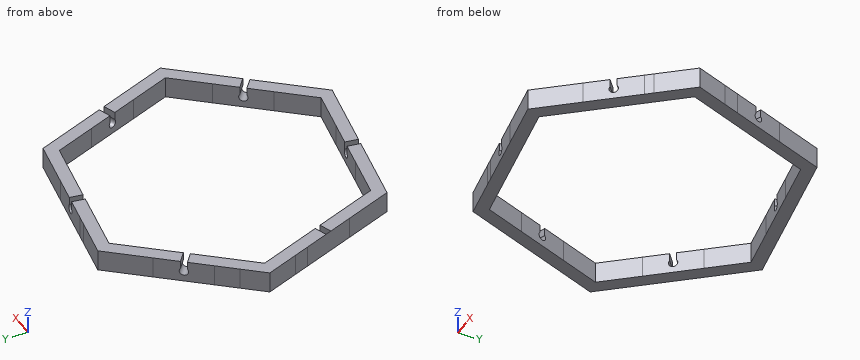
Autodesk Fusion 360 part; units mm, degrees
sketch "Sketch1" plane through (0, 0, 0) normal (0, 0, 1) x (1, 0, 0)
  line L0 (-10.798, 13.3938) -> (-13.526, 20.8958)
  line L1 (-9.4934, 25.6987) -> (-13.526, 20.8958)
  line L2 (19.2845, 47.1681) -> (9.9209, 48.822)
  line L3 (55.6112, 15.5789) -> (58.2905, 8.2107)
  line L4 (52.0708, 0.8027) -> (58.2905, 8.2107)
  line L5 (8.3931, -15.0435) -> (-1.0646, -13.373)
  line L6 (-10.798, 13.3938) -> (-9.5166, 9.87)
  line L7 (-5.074, -2.3473) -> (-1.0646, -13.373)
  line L8 (1.1628, -10.72) -> (-2.2546, -1.322)
  line L9 (-6.6972, 10.8953) -> (-10.1147, 20.2932)
  line L10 (33.6598, -16.4599) -> (23.8122, -14.7206)
  line L11 (11.0104, -12.4594) -> (1.1628, -10.72)
  line L12 (8.3931, -15.0435) -> (10.4886, -15.4136)
  line L13 (23.2904, -17.6748) -> (34.8436, -19.7155)
  line L14 (54.8793, 8.8133) -> (48.4491, 1.1547)
  line L15 (40.0899, -8.8014) -> (33.6598, -16.4599)
  line L16 (52.0708, 0.8027) -> (50.7467, -0.7743)
  line L17 (42.3875, -10.7304) -> (34.8436, -19.7155)
  line L18 (43.6017, 39.8265) -> (47.0192, 30.4285)
  line L19 (51.4618, 18.2112) -> (54.8793, 8.8133)
  line L20 (55.6112, 15.5789) -> (54.2812, 19.2364)
  line L21 (49.8385, 31.4537) -> (45.8292, 42.4795)
  line L22 (11.1048, 45.5664) -> (20.9523, 43.827)
  line L23 (33.7542, 41.5658) -> (43.6017, 39.8265)
  line L24 (19.2845, 47.1681) -> (21.4741, 46.7813)
  line L25 (34.276, 44.5201) -> (45.8292, 42.4795)
  line L26 (-10.1147, 20.2932) -> (-3.6845, 27.9518)
  line L27 (4.6746, 37.9079) -> (11.1048, 45.5664)
  line L28 (-9.4934, 25.6987) -> (-5.9821, 29.8808)
  line L29 (2.3771, 39.8369) -> (9.9209, 48.822)
  line L30 (50.7467, -0.7743) -> (42.3875, -10.7304)
  line L31 (40.0899, -8.8014) -> (48.4491, 1.1547)
  line L32 (23.2904, -17.6748) -> (10.4886, -15.4136)
  line L33 (11.0104, -12.4594) -> (23.8122, -14.7206)
  line L34 (-2.2546, -1.322) -> (-6.6972, 10.8953)
  line L35 (-9.5166, 9.87) -> (-5.074, -2.3473)
  line L36 (-3.6845, 27.9518) -> (4.6746, 37.9079)
  line L37 (2.3771, 39.8369) -> (-5.9821, 29.8808)
  line L38 (20.9523, 43.827) -> (33.7542, 41.5658)
  line L39 (34.276, 44.5201) -> (21.4741, 46.7813)
  line L40 (49.8385, 31.4537) -> (54.2812, 19.2364)
  line L41 (51.4618, 18.2112) -> (47.0192, 30.4285)
extrude "Extrude1" add sketch "Sketch1" along normal blind 5
sketch "Sketch2" plane through (8.6627, 49.0442, 0) normal (0.1739, 0.9848, 0) x (-0.9848, 0.1739, 0)
  line L0 (-37.7418, 0) -> (-1.2777, 0)
  line L1 (-1.2777, 0) -> (-1.2777, 5)
  line L2 (-1.2777, 5) -> (-37.7418, 5)
  line L3 (-37.7418, 5) -> (-37.7418, 0)
  line L4 (-20.2597, 5) -> (-20.2597, 3.1614)
  line L5 (-18.7597, 3.1614) -> (-18.7597, 5)
  arc A0 (-20.2597, 3.1614) -> (-18.7597, 3.1614) centre (-19.5097, 2.5) ccw
  arc A1 (-19.3816, 3.4918) -> (-19.5097, 3.5) centre (-19.5097, 2.5) ccw
  line L6 (-20.2597, 5) -> (-18.7597, 5)
  arc A2 (-20.2597, 3.1614) -> (-18.7597, 3.1614) centre (-19.5097, 2.5) ccw
  line L7 (-18.7597, 3.1614) -> (-18.7597, 5)
  line L8 (-20.2597, 5) -> (-20.2597, 3.1614)
  line L9 (-20.2597, 5) -> (-18.7597, 5)
  arc A3 (-20.2597, 3.1614) -> (-18.7597, 3.1614) centre (-19.5097, 2.5) ccw
  line L10 (-18.7597, 3.1614) -> (-18.7597, 5)
  line L11 (-20.2597, 5) -> (-20.2597, 3.1614)
  line L12 (-20.2597, 5) -> (-18.7597, 5)
  point P0 (-19.5097, 2.5)
  dimension "d30" = 2
  dimension "d34" = 2
  dimension "d35" = 2
sketch "Sketch3" plane through (-18.2237, 15.3006, 0) normal (-0.7659, 0.643, 0) x (-0.643, -0.7659, 0)
  line L0 (-43.7698, 0) -> (-7.3057, 0)
  line L1 (-7.3057, 0) -> (-7.3057, 5)
  line L2 (-7.3057, 5) -> (-43.7698, 5)
  line L3 (-43.7698, 5) -> (-43.7698, 0)
  arc A0 (-26.2597, 3.1614) -> (-24.7597, 3.1614) centre (-25.5097, 2.5) ccw
  line L4 (-24.7597, 3.1614) -> (-24.7597, 5)
  line L5 (-26.2597, 5) -> (-26.2597, 3.1614)
  line L6 (-26.2597, 5) -> (-24.7597, 5)
  dimension "d36" = 2
sketch "Sketch4" plane through (-5.2353, -1.9037, 0) normal (-0.9398, -0.3417, 0) x (0.3417, -0.9398, 0)
  line L0 (-24.2601, 0) -> (12.204, 0)
  line L1 (12.204, 0) -> (12.204, 5)
  line L2 (12.204, 5) -> (-24.2601, 5)
  line L3 (-24.2601, 5) -> (-24.2601, 0)
  arc A0 (-6.7597, 3.1614) -> (-5.2597, 3.1614) centre (-6.0097, 2.5) ccw
  line L4 (-5.2597, 3.1614) -> (-5.2597, 5)
  line L5 (-6.7597, 5) -> (-6.7597, 3.1614)
  line L6 (-6.7597, 5) -> (-5.2597, 5)
  dimension "d39" = 2
extrude "Extrude5" cut sketch "Sketch2" against normal blind 69 contours L2 L4 L5 A0 L6 A2 L7 L8 L9 A3 L10 L11 L12
extrude "Extrude6" cut sketch "Sketch3" against normal blind 67 contours L2 A0 L4 L5 L6
extrude "Extrude7" cut sketch "Sketch4" against normal blind 67 contours L2 A0 L4 L5 L6
Could you check a few things on this model? Use its own coordinates, in mm. Give positions to 0.01 mm unless a question says otherwise; leave off trailing zeros. Write each loop counter-clockwise with the first axis right and the second up, starting at its lowest first coordinate (ties: lowest second). Pieces come first, ordered by that corner, then holes. Notation, with made-up numbers: (82.5, 54) -> (102.5, 54) arc R20 ccw to (102.5, 85) -> close; hole circle Ø7 at (74, 78.25). An arc over 180 degrees is marked (long way). Answer as CSV lines item,"result". Start each with the question number.
(1) Please list where these lines run through material, in increasing order: line 1 (Y direction, x = 37.5, z = 3.4); line 2 (Y direction, x = 13.5, z = 1.5); line 3 (X direction, y = 17.5, z = 2.8).
(2) I'm going to push flat-ended pins straight in: pin 1 Ø1.5 at (y, z) = (24.5, 4.5) entering from +X; pin 2 Ø3 at (x, z) = (40.5, 4.5) entering from -Y; pin 3 Ø2 at (x, z) = (36, 2.5) entering from +Y. Where does each tip first touch, or does it pass through?
(3) If we section it at A-A, the plane x = 32: Write out the boundary of the cut face in (y, z).
(4) If we section it at B-B, the plane y = 37: Write out the boundary of the cut face in (x, z).
Answer list:
1,line 1,"-16.55 to -11.89, 40.9 to 43.95"
1,line 2,"-15.95 to -12.9, 45.14 to 48.19"
1,line 3,"-12.29 to -9.1, 51.72 to 54.91"
2,pin 1,"x = 52.64"
2,pin 2,"y = -14.77"
2,pin 3,"y = 44.39"
3,outline,"(-19.21, 0) -> (-16.17, 0) -> (-16.17, 5) -> (-19.21, 5) -> close; (41.88, 0) -> (44.92, 0) -> (44.92, 5) -> (41.88, 5) -> close"
4,outline,"(0, 0) -> (3.91, 0) -> (3.91, 5) -> (0, 5) -> close; (44.63, 0) -> (47.82, 0) -> (47.82, 5) -> (44.63, 5) -> close"
